Here's how the part is built. I have some questions about the finished solid (model axes, mm). Give positions to 0.01 mm unless a question says otherwise; leave off trailing zeros. Write each loop counter-clockwise with the first axis right and the second up, starting at its lowest first coordinate (ties: lowest second). Pieces come first, ordered by that corner, then holes. Notation, with made-up numbers: (-17.75, 21.25) - (23.25, 21.25) arc R16 ccw to (23.25, 42.25) - close; hole circle Ø6 at (48.25, 12). An arc over 180 degrees is marked (long way). Use one line per item in the form item = value. Start each with the question number.
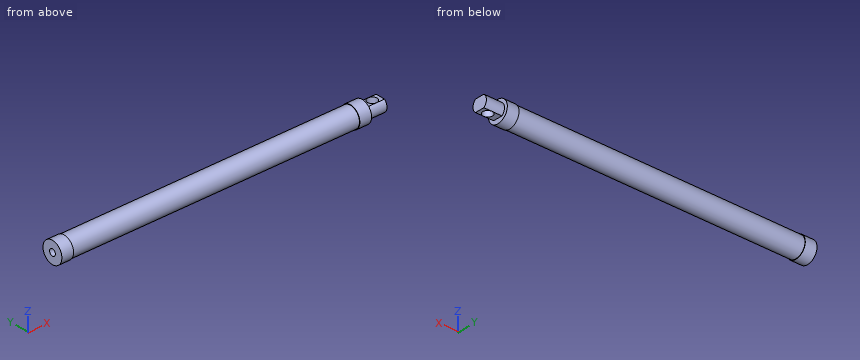
from build123d import *

# Parameters (mm, degrees)
SKETCH1_W               = 280
SKETCH1_H               = 9.58
CUT_EXTRUDE1_DEPTH      = 281.466018322
CUT_EXTRUDE1_DEPTH_BACK = 281.466018322
SKETCH2_R               = 3.05
SKETCH4_R               = 10
BOSS_EXTRUDE1_DEPTH     = 11
CUT_EXTRUDE2_DEPTH      = 281.500482539
CUT_EXTRUDE2_DEPTH_BACK = 281.500482539
SKETCH7_R               = 3.05
SKETCH11_R              = 10
BOSS_EXTRUDE2_DEPTH     = 11
CUT_EXTRUDE4_DEPTH      = 292.481595825
CUT_EXTRUDE4_DEPTH_BACK = 292.481595825
SKETCH12_R              = 3.05
SKETCH13_R              = 7.1
BOSS_EXTRUDE3_DEPTH     = 17
CUT_EXTRUDE5_DEPTH      = 178.977152858
CUT_EXTRUDE5_DEPTH_BACK = 178.977152858
SKETCH14_R              = 4.5
CUT_EXTRUDE6_REACH      = 310.455
SKETCH16_W              = 5.118750851
SKETCH16_H              = 10.923653892
SKETCH16_W_2            = 7.412502438


with BuildPart() as part:
    # Sketch1 → Revolve2 (revolve)
    with BuildSketch(Plane.XY, mode=Mode.PRIVATE) as revolve2_sk:
        with Locations((20.187319621, -1.354200627)):
            Rectangle(SKETCH1_W, SKETCH1_H)
    revolve(revolve2_sk.sketch.rotate(Axis((-119.812680379, 3.435799373, 0), (1, 0, 0)), 270), axis=Axis((-119.812680379, 3.435799373, 0), (1, 0, 0)))

    # Sketch2 → Cut-Extrude1 (cut, two sides: drawn at the far end of the back side and taken through both)
    with BuildSketch(Plane.ZY.offset(119.812680379).offset(-CUT_EXTRUDE1_DEPTH_BACK)):
        with Locations((0, 3.435799373)):
            Circle(SKETCH2_R)
    extrude(amount=CUT_EXTRUDE1_DEPTH + CUT_EXTRUDE1_DEPTH_BACK, mode=Mode.SUBTRACT)

    # Sketch4 → Boss-Extrude1 (add)
    with BuildSketch(Plane(origin=(160.187319621, 0, 0), x_dir=(0, 0, -1), z_dir=(1, 0, 0))):
        with Locations((0, 3.435799373)):
            Circle(SKETCH4_R)
    extrude(amount=-BOSS_EXTRUDE1_DEPTH)

    # Sketch7 → Cut-Extrude2 (cut, two sides: drawn at the far end of the back side and taken through both)
    with BuildSketch(Plane(origin=(160.187319621, 0, 0), x_dir=(0, 0, -1), z_dir=(1, 0, 0)).offset(-CUT_EXTRUDE2_DEPTH_BACK)):
        with Locations((0, 3.360575041)):
            Circle(SKETCH7_R)
    extrude(amount=CUT_EXTRUDE2_DEPTH + CUT_EXTRUDE2_DEPTH_BACK, mode=Mode.SUBTRACT)

    # Sketch11 → Boss-Extrude2 (add)
    with BuildSketch(Plane.ZY.offset(119.812680379)):
        with Locations((0, 3.360575041)):
            Circle(SKETCH11_R)
    extrude(amount=BOSS_EXTRUDE2_DEPTH)

    # Sketch12 → Cut-Extrude4 (cut, two sides: drawn at the far end of the back side and taken through both)
    with BuildSketch(Plane.ZY.offset(130.812680379).offset(-CUT_EXTRUDE4_DEPTH_BACK)):
        with Locations((0, 3.33623901)):
            Circle(SKETCH12_R)
    extrude(amount=CUT_EXTRUDE4_DEPTH + CUT_EXTRUDE4_DEPTH_BACK, mode=Mode.SUBTRACT)

    # Sketch13 → Boss-Extrude3 (add)
    with BuildSketch(Plane(origin=(160.187319621, 0, 0), x_dir=(0, 0, -1), z_dir=(1, 0, 0))):
        with Locations((0, 3.33623901)):
            Circle(SKETCH13_R)
    extrude(amount=BOSS_EXTRUDE3_DEPTH)

    # Sketch14 → Cut-Extrude5 (cut, two sides: drawn at the far end of the back side and taken through both)
    with BuildSketch(Plane.XY.offset(-CUT_EXTRUDE5_DEPTH_BACK)):
        with Locations((169.687319621, 3.33623901)):
            Circle(SKETCH14_R)
    extrude(amount=CUT_EXTRUDE5_DEPTH + CUT_EXTRUDE5_DEPTH_BACK, mode=Mode.SUBTRACT)

    # Cut-Extrude6: up to this face of the body (flat: up to its plane)
    cut_extrude6_end = Plane(part.part.faces().sort_by_distance((160.187319621, 3.435799373, 9.717157288))[0])
    # Sketch16 → Cut-Extrude6 (cut, up to the picked face)
    with BuildSketch(Plane(origin=(177.187319621, 0, 0), x_dir=(0, 0, -1), z_dir=(1, 0, 0)), mode=Mode.PRIVATE) as cut_extrude6_sk1:
        with Locations((-8.074815219, 2.345421333)):
            Rectangle(SKETCH16_W, SKETCH16_H)
    cut_extrude6_tool1 = split(extrude(cut_extrude6_sk1.sketch, amount=-CUT_EXTRUDE6_REACH, mode=Mode.PRIVATE), bisect_by=cut_extrude6_end, keep=Keep.BOTH, mode=Mode.PRIVATE)
    # Sketch16 → Cut-Extrude6 (cut, up to the picked face)
    with BuildSketch(Plane(origin=(177.187319621, 0, 0), x_dir=(0, 0, -1), z_dir=(1, 0, 0)), mode=Mode.PRIVATE) as cut_extrude6_sk2:
        with Locations((9.221691013, 2.345421333)):
            Rectangle(SKETCH16_W_2, SKETCH16_H)
    cut_extrude6_tool2 = split(extrude(cut_extrude6_sk2.sketch, amount=-CUT_EXTRUDE6_REACH, mode=Mode.PRIVATE), bisect_by=cut_extrude6_end, keep=Keep.BOTH, mode=Mode.PRIVATE)
    add(cut_extrude6_tool1.solids().sort_by(Axis((177.18732, 2.345421, 8.074815), (-1, 0, 0)))[0], mode=Mode.SUBTRACT)
    add(cut_extrude6_tool2.solids().sort_by(Axis((177.18732, 2.345421, -9.221691), (-1, 0, 0)))[0], mode=Mode.SUBTRACT)


solid = part.part
1. I want a section at A-A, the plane z = 0. List the corners of the cut face in (x, y) for me, then the cut area to 3 significant figures.
2. Please list where these lines run through material, in increasing order: line 1 (Z direction, x = 49.5, y = 3.25); line 2 (Y direction, x = -4.5, z = 0.5); line 3 (X direction, y = 5.5, z = -9).
3. For P1, Ø4, axis at x = -32.5, z = -8, coming from the +Y side; P2, Ø8, axis at x = 169.69, y = 3.34, coming from the -Z side; P3, Ø3.5, axis at x = 172.5, y = 5.5, coming from the +Z side; P4, Ø5, axis at y = -4, z = 6.5, coming from the +X side, each with a flat end and sliding along its axis, tell me the tip position at first contact or that it passes through.
4. I want a section at B-B, the plane x = -67.5. List the corners of the cut face in (y, z) for me.
Result sheet:
q1.outline = (-130.81, -6.64) - (-119.81, -6.64) - (-119.81, -6.14) - (149.19, -6.14) - (149.19, -6.56) - (160.19, -6.56) - (160.19, -3.76) - (177.19, -3.76) - (177.19, 10.44) - (160.19, 10.44) - (160.19, 13.44) - (149.19, 13.44) - (149.19, 13.02) - (-119.81, 13.02) - (-119.81, 13.36) - (-130.81, 13.36) - (-130.81, 6.39) - (-119.81, 6.39) - (-119.81, 6.49) - (149.19, 6.49) - (149.19, 6.41) - (160.19, 6.41) - (160.19, 0.29) - (-130.81, 0.29) - close; hole circle Ø9 at (169.69, 3.34)
q1.area = 3,970 mm2
q2.line_1 = -9.58 to -3.05, 3.05 to 9.58
q2.line_2 = -6.13 to 0.33, 6.44 to 13
q2.line_3 = -130.81 to 160.19
q3.P1 = 10.9
q3.P2 = through
q3.P3 = 5.52
q3.P4 = 160.19
q4.outline = circle Ø19.16 at (3.44, 0); hole (3.35, -3.05) arc R3.05 ccw to (3.4, -3.05) arc R3.05 ccw (long way) to (3.4, 3.05) arc R3.05 ccw to (3.35, 3.05) arc R3.05 ccw (long way) to start
